```python
from build123d import *

# Parameters (mm, degrees)
F1_DEPTH       = 3
F3_D           = 3.3
F3_DEPTH       = 14.4
F3_CBORE_D     = 6.5
F3_CBORE_DEPTH = 3
F3_TIP         = 0.9914200214


# Not quite as in the source:
# - a feature names something its author has since deleted; it is built from what else it names


with BuildPart() as f1:
    # F0 (on Front) → F1 (new body)
    with BuildSketch(Plane.XZ):
        with BuildLine():
            Line((52.4541210128, 6.1781848239), (-19.9804399163, 6.1781848239))
            Line((-19.9804399163, 6.1781848239), (-19.9804399163, -14.0438194092))
            Line((-19.9804399163, -14.0438194092), (52.5663935712, -14.0438194092))
            ThreePointArc((52.5663935712, -14.0438194092), (61.0848860922, -9.2816896986), (61.4901453485, 0.469123557))
            Line((61.4901453485, 0.469123557), (61.3778727901, 0.6911277901))
            ThreePointArc((61.3778727901, 0.6911277901), (57.6919913022, 4.696677345), (52.4541210128, 6.1781848239))
        make_face()
    extrude(amount=F1_DEPTH)

    # F3
    with Locations(Plane.XZ.offset(3)):
        with Locations((36.2392867059, -6.078066061), (6.7392867059, -6.1909663491)):
            CounterBoreHole(F3_D / 2, F3_CBORE_D / 2, F3_CBORE_DEPTH, depth=F3_DEPTH)
            with Locations((0, 0, -(F3_DEPTH + F3_TIP / 2))):  # 118° drill point
                Cone(0, F3_D / 2, F3_TIP, mode=Mode.SUBTRACT)


solid = f1.part
```
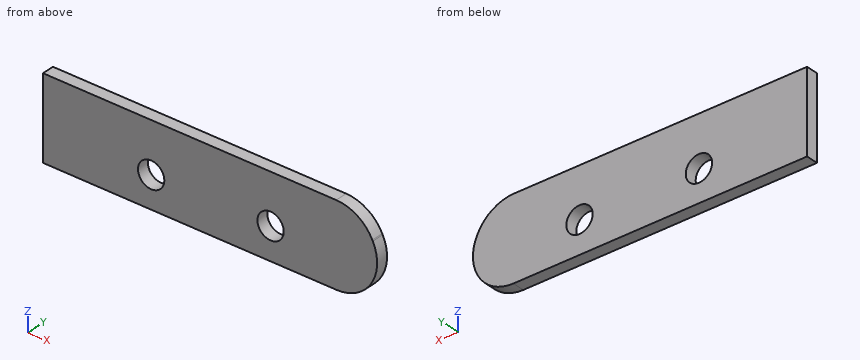
Here's how the part is built. I have some questions about the finished solid (model axes, mm). Coordinates: 2 decimals unless noted, no trailing zeros. Order: outer loops, then holes, each group sorted by start corner. A loop starts at its lowest first (then second) coordinate and runs counter-clockwise, first axis right, second up. Notation, with made-up numbers: (77, 57.25) - (126, 57.25) arc R20 cw to (126, 95.25) - close; hole circle Ø3 at (44.5, -33). An arc over 180 degrees is marked (long way). One line per question, with ' | ' between items.
(1) Suppose I cut it at C-C on z = 3. List the corners of the cut face in (x, y) for me.
Report:
outline: (-19.98, -3) - (59.77, -3) - (59.77, 0) - (-19.98, 0) - close
(2) If I drill on L1, parallel to X at y = -0.4, z = -7; L2, parallel to Z at x = 5, y = -1.45; L3, parallel to X at y = -0.8, z = -6.5, over which ranges is the centre line in solid material (lowest first)?
Report:
L1: x = -19.98 to 3.59, 9.89 to 33.12, 39.36 to 62.12 | L2: z = -14.04 to -8.94, -3.45 to 6.18 | L3: x = -19.98 to 3.5, 9.97 to 33.02, 39.46 to 62.26
(3) Suppose I cut it at A-A on z = -8.5. List the corners of the cut face in (x, y) for me, and give its area (3 significant figures).
Report:
outline: (-19.98, -3) - (4.45, -3) - (4.45, 0) - (-19.98, 0) - close; (9.03, -3) - (34.07, -3) - (34.07, 0) - (9.03, 0) - close; (38.41, -3) - (61.52, -3) - (61.52, 0) - (38.41, 0) - close | area: 218 mm2
(4) Suppose I cut it at B-B on y = -1.85. List the corners of the cut face in (x, z) for me, and give its area (3 significant figures).
Report:
outline: (-19.98, -14.04) - (52.57, -14.04) arc R10 ccw to (61.49, 0.47) - (61.38, 0.69) arc R10 ccw to (52.45, 6.18) - (-19.98, 6.18) - close; hole circle Ø6.5 at (6.74, -6.19); hole circle Ø6.5 at (36.24, -6.08) | area: 1,560 mm2
(5) Will these pins go through, and if not, where does the flat tip stop? pin 1 (7.5 mm diameter, centred on x = 36.24, z = -6.08, fed in from +Y); pin 2 (1 mm diameter, centred on y = -2, z = -2, fed in from +X); pin 3 (4 mm diameter, centred on x = 6.74, z = -6.19, fed in from -Y).
Report:
pin 1: stops at y = 0 | pin 2: stops at x = 62.45 | pin 3: passes through
(6) Suppose I cut it at D-D on z = -12.5. List the corners of the cut face in (x, y) for me, and give its area (3 significant figures).
Report:
outline: (-19.98, -3) - (57.9, -3) - (57.9, 0) - (-19.98, 0) - close | area: 234 mm2
